Read the model definition and answer for the solid it produces. Units are mm, in the model's axes. Face numbers are marked on the shaded views. Coordinates: 2 decimals unless noted, no trailing zeros. Loops run counter-clockwise (first coordinate to the right, second up) from the corner with the lowest first, then second, coordinate; pieces in that order, holes last. Notation, with made-up numbers: (21.5, -5.75) - (45.5, -5.75) arc R27 ccw to (45.5, 22.25) - close; hole circle Ø6 at (66.25, 0). An arc over 180 degrees is marked (long way). One line per item, written item: value. Start each with the question number.
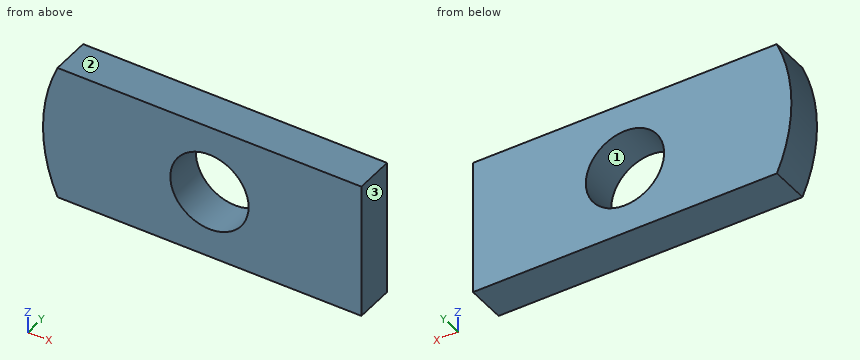
from build123d import *

# Parameters (mm, degrees)
F0_R     = 1.5875
F1_DEPTH = 0.8001


with BuildPart() as f1:
    # F0 (on Front) → F1 (new body, symmetric)
    with BuildSketch(Plane.XZ):
        with BuildLine():
            Line((6.240089, 2.755591), (-6.083732, 2.755591))
            ThreePointArc((-6.083732, 2.755591), (-6.671816, 0), (-6.083732, -2.755591))
            Line((-6.083732, -2.755591), (6.240089, -2.755591))
            Line((6.240089, -2.755591), (6.240089, 2.755591))
        make_face()
        with Locations((0.078179, 0)):
            Circle(F0_R, mode=Mode.SUBTRACT)
    extrude(amount=F1_DEPTH, both=True)


solid = f1.part
1) Straight lines are drawn through the part: L1, parallel to X at y = 0.6, z = -0.1; L2, parallel to X at y = 0.7, z = 0.85; L3, parallel to X at y = 0.5, z = -1.8. For each, find the intervals that lie inside material, in ascending order.
2) Section D-D, the plane z = -1.95 is taken. Determine the outline of the cut face in (x, y), and give its area (3 significant figures).
3) Section B-B, the plane x = 1.25 is taken. Determine the outline of the cut face in (y, z).
4) Determine the mould class of the marked faces 1, 2 and 3 for opening direction Z: released by +Z, released by -Z, zero draft, split by the parting line, or undercut.
5) Section A-A, the plane z = 0 is taken. Determine the outline of the cut face in (x, y).
Answer below:
1. L1: -6.67 to -1.51, 1.66 to 6.24
1. L2: -6.62 to -1.26, 1.42 to 6.24
1. L3: -6.43 to 6.24
2. outline: (-6.38, -0.8) - (6.24, -0.8) - (6.24, 0.8) - (-6.38, 0.8) - close
2. area: 20.2 mm2
3. outline: (-0.8, -2.76) - (0.8, -2.76) - (0.8, -1.07) - (-0.8, -1.07) - close; (-0.8, 1.07) - (0.8, 1.07) - (0.8, 2.76) - (-0.8, 2.76) - close
4. face 1: undercut
4. face 2: released by +Z
4. face 3: zero draft
5. outline: (-6.67, -0.8) - (-1.51, -0.8) - (-1.51, 0.8) - (-6.67, 0.8) - close; (1.67, -0.8) - (6.24, -0.8) - (6.24, 0.8) - (1.67, 0.8) - close
